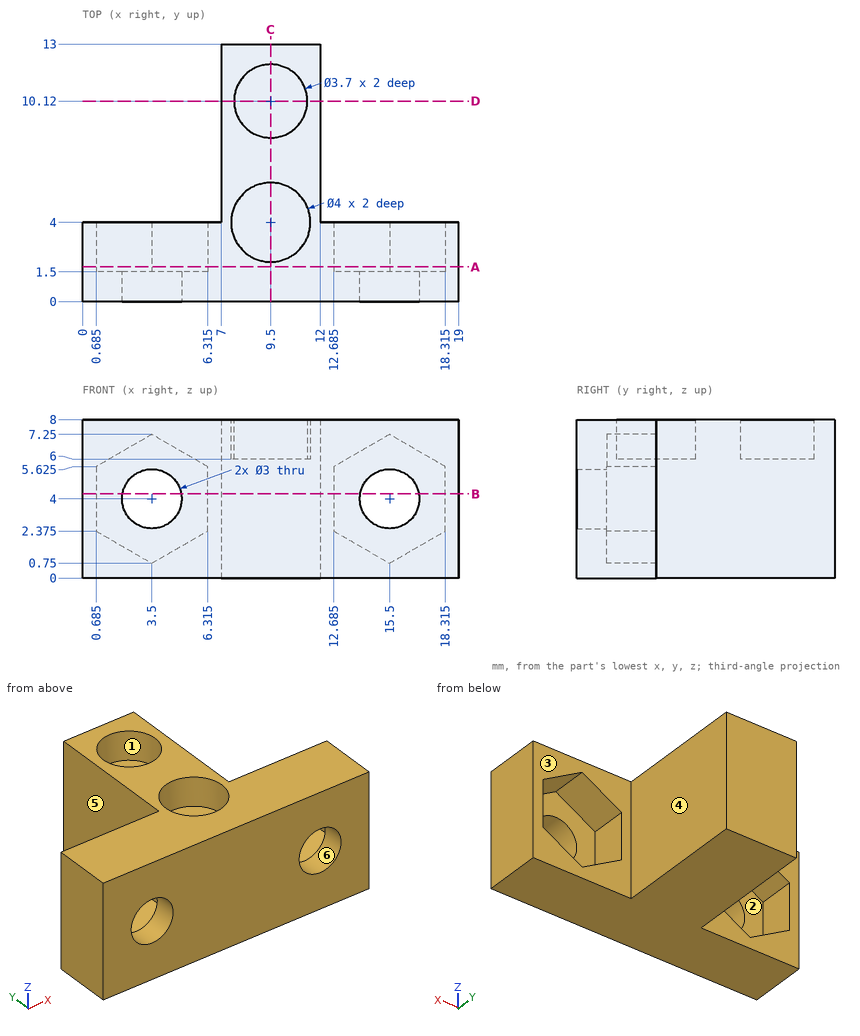
Could you check a few things on this drawing? It's one solid part, dimensions in mm from its lowest x, y, z. A direction names the side the tool comes from. Coordinates: 2 decimals unless noted, no trailing zeros. Write each loop counter-clockwise with the first axis right and the second up, starting at its lowest first coordinate (ties: lowest second). Pieces come first, ordered by that corner, then holes. Notation, with made-up numbers: (-37.75, -33) - (-4.75, -33) arc R23 ccw to (-4.75, -8) - close; hole circle Ø4 at (-39, 16.5). An arc over 180 degrees is marked (long way). Put each result on its own line as item: value. Start each with the question number.
Q1. I want a section at B-B on z = 4.25. Write out the boundary of the cut face in (x, y) (1 decimal).
Q2. I want a section at C-C on x = 9.5. Write out the boundary of the cut face in (y, z), plus the area to 3 significant figures.
Q3. Thinking about a two-plate mould opening in X: for the marked faces 4, 5 and 6, which applies, pulls with the +X half, pulls with the -X half, needs draft (parallel to the pull), parting line crosses it, or undercut?
Q4. I'm going to push flat-ended pins straight in: P1, Ø1.5, axis at y = 11, z = 1.5, coming from the -X side; P2, Ø2.5, axis at x = 9.5, y = 4, coming from the +Z side; P3, Ø2, axis at y = 4.5, z = 1.5, coming from the +X side; P4, Ø2, axis at x = 4.5, z = 3, coming from the +Y side. Where does each tip first touch, or does it pass through?
Q5. Which directions (+Z, -Z, +X, -X, +Y, -Y) give clear straight access to the entire face, cutting with the end or side of a thin tool? Please do the marked faces 1, 2 and 3.
Q6. I want a section at D-D on y = 10.12. Write out the boundary of the cut face in (x, z).
Q7. Please list where these lines run through material, in increasing order: L1, parallel to Y at x = 9.5, z = 7.6; L2, parallel to X at y = 1, z = 4; L3, parallel to Z at x = 3.5, y = 0.4.
Q8. I want a section at A-A on y = 1.75. Count the separate pieces of the cut face and the enclosed holes in it.
Checks:
1. outline: (0, 0) - (2, 0) - (2, 1.5) - (0.7, 1.5) - (0.7, 4) - (0, 4) - close; (5, 0) - (14, 0) - (14, 1.5) - (12.7, 1.5) - (12.7, 4) - (12, 4) - (12, 13) - (7, 13) - (7, 4) - (6.3, 4) - (6.3, 1.5) - (5, 1.5) - close; (17, 0) - (19, 0) - (19, 4) - (18.3, 4) - (18.3, 1.5) - (17, 1.5) - close
2. outline: (0, 0) - (13, 0) - (13, 8) - (11.97, 8) - (11.97, 6) - (8.27, 6) - (8.27, 8) - (6, 8) - (6, 6) - (2, 6) - (2, 8) - (0, 8) - close
2. area: 88.6 mm²
3. face 4: pulls with the +X half
3. face 5: pulls with the -X half
3. face 6: undercut
4. P1: x = 7
4. P2: z = 6
4. P3: x = 19
4. P4: y = 1.5
5. face 1: +Z
5. face 2: +Y
5. face 3: +Z, -Z, +X, +Y
6. outline: (7, 0) - (12, 0) - (12, 8) - (11.35, 8) - (11.35, 6) - (7.65, 6) - (7.65, 8) - (7, 8) - close
7. L1: 0 to 2, 6 to 8.27, 11.97 to 13
7. L2: 0 to 2, 5 to 14, 17 to 19
7. L3: 0 to 2.5, 5.5 to 8
8. separate pieces: 1
8. enclosed holes: 2
